Part model, mm, in its own coordinate system. Face numbers are marked on the shaded views. A direction names the side the tool comes from. Round coordinates to 2 decimals unless told otherwise and drop trailing zeros. Write each loop counter-clockwise with the first axis right and the second up, starting at its lowest first coordinate (ties: lowest second). Pieces come first, ordered by that corner, then holes. Notation, with made-up numbers: M 5,-7 L 17,-7 A23 cw 17,30 Z; hole C 39,64 d5. An arc over 180 degrees is marked long. Use a Markdown table: item, result. Add a question column.
1) Slice it at B-B on x = 70. Write the cut outline in (y, z), plus the area to 3 significant figures.
2) Slice it at C-C on y = 57. Write the cut outline in (x, z).
3) Slice it at A-A on z = 0. Give the number of separate pieces and of enclosed holes in the cut face, plus the area to 3 significant figures.
4) Which spindle directions (+Z, -Z, +X, -X, +Y, -Y) get a long thin tool onto all of the face, cutting with end or side? Do the marked faces 1 and 2. Say none if no direction does.
5) Drop flat-ended pins along their axis: P1, Ø12, axis at x = 43.5, z = 6, coming from the +Y side; P2, Ø13, axis at x = 68.26, z = 0, coming from the -Y side; P3, Ø1, axis at y = 13.5, z = -11, coming from the +X side. Give the stop position or say it passes through.
6) Wall check: probe 1 along X at (y, z) = (2.5, 0); probe 2 along X at (y, z) = (79.5, -18). Give the ranges that are in metal, low to high.
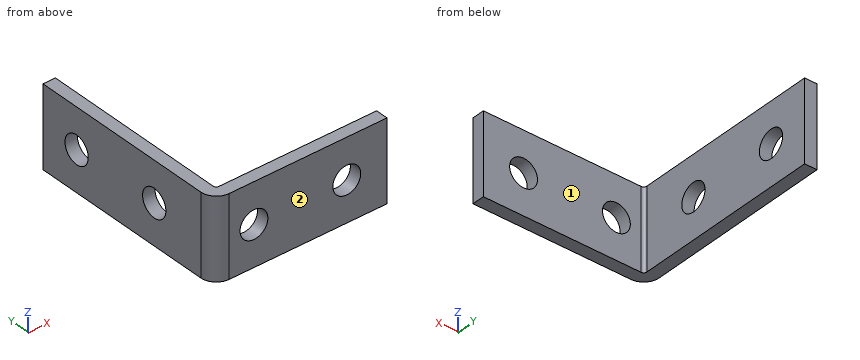
```python
from build123d import *

# Parameters (mm, degrees)
EXTRUDE_THIN1_DEPTH = 20.6375
SKETCH2_R           = 7.14375
CUT_EXTRUDE1_DEPTH  = 135.225917882
SKETCH3_R           = 7.14375
CUT_EXTRUDE2_DEPTH  = 135.974847773


with BuildPart() as part:
    # Sketch1 → Extrude-Thin1 (new, symmetric)
    with BuildSketch(Plane.XY):
        with BuildLine():
            Line((0, 104.775), (0, 7.9375))
            ThreePointArc((0, 7.9375), (2.324839924, 2.324839924), (7.9375, 0))
            Line((7.9375, 0), (88.9, 0))
            Line((88.9, 0), (88.9, 6.35))
            Line((88.9, 6.35), (7.9375, 6.35))
            ThreePointArc((7.9375, 6.35), (6.814967985, 6.814967985), (6.35, 7.9375))
            Line((6.35, 7.9375), (6.35, 104.775))
            Line((6.35, 104.775), (0, 104.775))
        make_face()
    extrude(amount=EXTRUDE_THIN1_DEPTH, both=True)

    # Sketch2 → Cut-Extrude1 (cut, through all)
    with BuildSketch(Plane(origin=(0, 6.35, 0), x_dir=(1, 0, 0), z_dir=(0, 1, 0))):
        with Locations(Location((68.2625, 0, 0), (0, 0, 270))):
            Circle(SKETCH2_R)
        with Locations(Location((20.6375, 0, 0), (0, 0, 270))):
            Circle(SKETCH2_R)
    extrude(amount=-CUT_EXTRUDE1_DEPTH, mode=Mode.SUBTRACT)

    # Sketch3 → Cut-Extrude2 (cut, through all)
    with BuildSketch(Plane(origin=(6.35, 0, 0), x_dir=(0, 0, -1), z_dir=(1, 0, 0))):
        with Locations(Location((0, 84.1375, 0), (0, 0, 90))):
            Circle(SKETCH3_R)
        with Locations(Location((0, 36.5125, 0), (0, 0, 90))):
            Circle(SKETCH3_R)
    extrude(amount=-CUT_EXTRUDE2_DEPTH, mode=Mode.SUBTRACT)


solid = part.part
```
Entries:
| question | item | result |
|---|---|---|
| 1 | outline | M 0,-20.64 L 6.35,-20.64 L 6.35,-6.93 L 0,-6.93 Z; M 0,6.93 L 6.35,6.93 L 6.35,20.64 L 0,20.64 Z |
| 1 | area | 174 mm^2 |
| 2 | outline | M 0,-20.64 L 6.35,-20.64 L 6.35,20.64 L 0,20.64 Z |
| 3 | separate pieces | 5 |
| 3 | enclosed holes | 0 |
| 3 | area | 814 mm^2 |
| 4 | face 1 | +Z, -Z, +X, +Y |
| 4 | face 2 | +Z, -Z, +X, -X, -Y |
| 5 | P1 | stops at y = 6.35 |
| 5 | P2 | passes through |
| 5 | P3 | stops at x = 6.35 |
| 6 | probe 1 | x = 2.15 to 13.49, 27.78 to 61.12, 75.41 to 88.9 |
| 6 | probe 2 | x = 0 to 6.35 |
